Here's how the part is built. I have some questions about the finished solid (model axes, mm). A direction names the side the tool comes from. Coordinates: 2 decimals unless noted, no trailing zeros. Loops run counter-clockwise (first coordinate to the right, second up) from the corner with the lowest first, then second, coordinate; pieces in that order, holes last. Notation, with made-up numbers: M 53.25,78.5 L 80.25,78.5 A29 cw 80.25,99.5 Z; hole C -15.5,-26 d7. An arc over 180 degrees is marked long. Use one line per item in the form item = value. Start each with the question number.
(1) Imagine slicing it at B-B, the plane z = 0. Please give me the cut outline in (x, y).
(2) Imagine slicing it at D-D, the plane y = -6. State how many separate pieces and enclosed holes the cut face has, and give its area (3 significant figures).
(3) Thinking about a two-plate mould opening in Z: for faces 1 (the flat face through (0, -4, 0)), 2 (the flat face through (2, 4, 4)), 3 (the cylindrical face through (4.056, -13.887, -10.648)), 4 (the cylindrical face through (4, 3, 0)), which applies, +Z half, -Z half, draft (parallel to the pull), parting line (faces both ways), or undercut?
(4) Imagine slicing it at A-A, the plane y = 0. Please give me the cut outline in (x, z).
(5) Imagine slicing it at C-C, the plane x = 3.5. Please give me the cut outline in (y, z), and give its area (3 significant figures).
(6) Please list where these lines run through material, in increasing order: L1, parallel to Z at x = 0.75, y = 0; L2, parallel to Z at x = 5.5, y = 0; L3, parallel to Y at x = 1.75, z = -9.
(7) On a 3-axis mill with a long thin cutter (end or side, diameter ignored), from which of +Z, -Z, +X, -X, +Y, -Y can I reach the whole of each face in a straight line? I mean faces 5 (the cylindrical face through (5.04, 1.08, 4.88)), 6 (the cylindrical face through (1.014, 4.74, -11.925)). Say none if no direction works.
(8) Will these pins go through, and if not, where does the flat tip stop? P1, Ø3, axis at x = 3.5, z = -3, coming from the +Y side; P2, Ø3, axis at y = -13, z = 11, coming from the -X side; P3, Ø5, axis at y = -5.88, z = -8.09, coming from the +X side; P4, Ø4, axis at x = 5, z = -3, coming from the -Y side.
```python
from build123d import *

# Parameters (mm, degrees)
F0_W            = 8
F0_H            = 17.5
F3_D            = 6
F4_T            = -2
F6_D            = 8
F6_COPIES_COUNT = 5
F7_SIZE         = 1


# Not quite as in the source:
# - a pattern or mirror of a feature is missing from the dataset's text; its kind, count and spacing are read off the source's solid


with BuildPart() as f1:
    # F0 (on Top) → F1 (revolve)
    with BuildSketch(Plane.XY):
        with Locations((4, 8.75)):
            Rectangle(F0_W, F0_H)
    revolve(axis=Axis((4, 0, 0), (1, 0, 0)))

    # F3 (through all)
    with Locations(Plane(origin=(0, 0, 0), x_dir=(0, 1, 0), z_dir=(-1, 0, 0))):
        with Locations((0, 0)):
            Hole(F3_D / 2)

    # F4
    f4_openings = [f1.faces().sort_by_distance(p)[0] for p in [
        (8, -17.005025, 0),
    ]]
    offset(amount=F4_T, openings=f4_openings)

    # F6 (through all)
    with Locations(Plane(origin=(0, 0, 0), x_dir=(0, 1, 0), z_dir=(-1, 0, 0))):
        with Locations((0, -10)):
            f6 = Hole(F6_D / 2)

    # F6_copies: F6 ×5 about axis
    f6_copies_axis = Axis((0, 0, 0), (1, 0, 0))
    for i in range(1, F6_COPIES_COUNT):
        add(f6.rotate(f6_copies_axis, i * 360 / F6_COPIES_COUNT), mode=Mode.SUBTRACT)

    # F7
    f7_edges = [f1.edges().sort_by_distance(p)[0] for p in [
        (8, -15.5, 0),
    ]]
    chamfer(f7_edges, length=F7_SIZE)


solid = f1.part
```
Answer:
q1.outline = M 0,-17.5 L 8,-17.5 L 8,-16.5 L 7,-15.5 L 2,-15.5 L 2,-12.05 L 0,-12.05 Z; M 0,-6.97 L 2,-6.97 L 2,-5 L 8,-5 L 8,-3 L 0,-3 Z; M 0,3 L 8,3 L 8,5 L 2,5 L 2,6.97 L 0,6.97 Z; M 0,12.05 L 2,12.05 L 2,15.5 L 7,15.5 L 8,16.5 L 8,17.5 L 0,17.5 Z
q2.separate_pieces = 3
q2.enclosed_holes = 0
q2.area = 66.8 mm²
q3.face_1 = draft
q3.face_2 = undercut
q3.face_3 = parting line
q3.face_4 = undercut
q4.outline = M 0,-17.5 L 8,-17.5 L 8,-16.5 L 7,-15.5 L 2,-15.5 L 2,-5 L 8,-5 L 8,-3 L 0,-3 Z; M 0,3 L 8,3 L 8,5 L 2,5 L 2,6 L 0,6 Z; M 0,14 L 2,14 L 2,15.5 L 7,15.5 L 8,16.5 L 8,17.5 L 0,17.5 Z
q5.outline = C 0,0 d35; C 0,0 d10; hole C 0,0 d31; hole C 0,0 d6
q5.area = 258 mm²
q6.L1 = -17.5 to -3, 3 to 6, 14 to 17.5
q6.L2 = -17.5 to -15.5, -5 to -3, 3 to 5, 15.5 to 17.5
q6.L3 = -15.01 to -9.77, -1.98 to 1.98, 9.77 to 15.01
q7.face_5 = +X
q7.face_6 = +X, -X
q8.P1 = 17.44
q8.P2 = 0
q8.P3 = through
q8.P4 = -17.47
